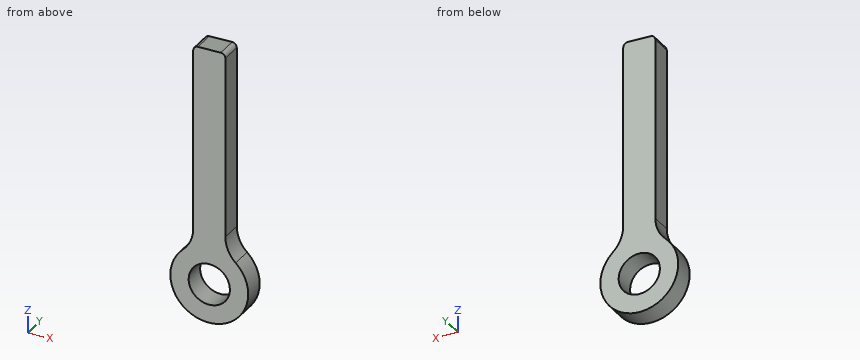
```python
from build123d import *

# Parameters (mm, degrees)
ESBO_O1_R          = 4.5
FLANGE_BASE1_DEPTH = 4.8


# Sheet-metal steps are written as plain solids
with BuildPart() as part:
    # Esboço1 → Flange-base1 (new body)
    with BuildSketch(Plane(origin=(0, 0, 0), x_dir=(1, 0, 0), z_dir=(0, 1, 0))):
        with BuildLine():
            Line((-3.5, 40.598245749), (-3.5, 1))
            ThreePointArc((-3.5, 1), (-3.207106781, 0.292893219), (-2.5, 0))
            Line((-2.5, 0), (2.5, 0))
            ThreePointArc((2.5, 0), (3.207106781, 0.292893219), (3.5, 1))
            Line((3.5, 1), (3.5, 40.598245749))
            ThreePointArc((3.5, 40.598245749), (4.089323422, 43.4095134), (5.758064516, 45.747425088))
            ThreePointArc((5.758064516, 45.747425088), (0, 60.5), (-5.758064516, 45.747425088))
            ThreePointArc((-5.758064516, 45.747425088), (-4.089323422, 43.4095134), (-3.5, 40.598245749))
        make_face()
        with Locations(Location((0, 52, 0), (0, 0, 270))):
            Circle(ESBO_O1_R, mode=Mode.SUBTRACT)
    extrude(amount=-FLANGE_BASE1_DEPTH)


solid = part.part
```
Check sheet for the modelled part. Datum: model origin and axes. Units: mm. Coordinates: 2 decimals unless noted, no trailing zeros. Write each loop counter-clockwise with the first axis right and the second up, starting at its lowest first coordinate (ties: lowest second). Pieces come first, ordered by that corner, then holes. Notation, with made-up numbers: M -21,47.25 L 34,47.25 A21 ccw 34,52.25 Z; hole C 68,-34 d11. An arc over 180 degrees is marked long. Use one line per item in the form item = value.
Item 1: Sectioned sample at C-C, the plane z = -52. Record the cut outline in (x, y), and give its area (3 significant figures).
Answer below:
outline = M -8.5,-4.8 L -4.5,-4.8 L -4.5,0 L -8.5,0 Z; M 4.5,-4.8 L 8.5,-4.8 L 8.5,0 L 4.5,0 Z
area = 38.4 mm^2
Item 2: Sectioned sample at A-A, the plane y = -3.7. Record the cut outline in (x, z), and give its area (3 significant figures).
Answer below:
outline = M -5.76,-45.75 A8.5 ccw long 5.76,-45.75 A7 cw 3.5,-40.6 L 3.5,-1 A1 ccw 2.5,0 L -2.5,0 A1 ccw -3.5,-1 L -3.5,-40.6 A7 cw Z; hole C 0,-52 d9
area = 473 mm^2
Item 3: Material ranges on L1, parallel to X at y = -2.5, z = -52; L2, parallel to X at y = -2.15, z = -30.5; L3, parallel to Z at x = -2.25, y = -3.7, recorded low to high. Write a range as from..to.
Answer below:
L1 = -8.5..-4.5, 4.5..8.5
L2 = -3.5..3.5
L3 = -60.2..-55.9, -48.1..0
Item 4: Sectioned sample at B-B, the plane x = 0. Record the cut outline in (y, z), and give its area (3 significant figures).
Answer below:
outline = M -4.8,-60.5 L 0,-60.5 L 0,-56.5 L -4.8,-56.5 Z; M -4.8,-47.5 L 0,-47.5 L 0,0 L -4.8,0 Z
area = 247 mm^2
Item 5: Gauge pin test, flat ends, axial feed: pin 1 Ø1 at (x, y) = (1, -3) entering from -Z; pin 2 Ø1.4 at (y, z) = (-2, -17) entering from +X; pin 3 Ø1.5 at (x, z) = (-5, -15.5) entering from -Y; pin 4 Ø2.5 at (y, z) = (-3, -18.5) entering from -X. Record the tip position at first contact, or that the pin passes through.
Answer below:
pin_1 = -60.49
pin_2 = 3.5
pin_3 = through
pin_4 = -3.5
Item 6: Sectioned sample at D-D, the plane z = -6.5. Record the cut outline in (x, y).
Answer below:
outline = M -3.5,-4.8 L 3.5,-4.8 L 3.5,0 L -3.5,0 Z
